Autodesk Inventor part; units mm, degrees
ref_plane "YZ Plane" through (0, 0, 0) normal (1, 0, 0) x (0, 1, 0)
ref_plane "XZ Plane" through (0, 0, 0) normal (0, 1, 0) x (-1, 0, 0)
ref_plane "XY Plane" through (0, 0, 0) normal (0, 0, 1) x (1, 0, 0)
sketch "Sketch1" plane through (0, 0, 0) normal (0, 0, 1) x (1, 0, 0)
  line L0 (-216.5289, 82.2753) -> (-216.5289, 432.2753)
  line L1 (-216.5289, 432.2753) -> (283.4711, 432.2753)
  line L2 (283.4711, 432.2753) -> (283.4711, 82.2753)
  arc A0 (-216.5289, 82.2753) -> (283.4711, 82.2753) centre (33.4711, 82.2753) ccw
  point P0 (0, 0)
  dimension "d0" = 500
  dimension "d1" = 250
  dimension "d2" = 350
extrude "Extrusion1" add sketch "Sketch1" against normal blind 1000
shell "Shell1" thickness 20 removed faces 1 at (-49.8623, 432.2753, -333.3333)
ref_plane "Work Plane1" through (-216.5289, -262.4747, 0) normal (0, 1, 0) x (-1, 0, 0)
sketch "Sketch2" plane through (-216.5289, -262.4747, 0) normal (0, 1, 0) x (-1, 0, 0)
  point P0 (-216.5289, 0)
sketch "Sketch3" plane through (-216.5289, -262.4747, 0) normal (0, 1, 0) x (-1, 0, 0)
  line L0 (-110, -915) -> (-30, -915)
  line L1 (-30, -915) -> (-30, -835)
  line L2 (-30, -835) -> (-110, -835)
  line L3 (-110, -835) -> (-110, -915)
  line L4 (-390, -915) -> (-470, -915)
  line L5 (-470, -915) -> (-470, -835)
  line L6 (-470, -835) -> (-390, -835)
  line L7 (-390, -835) -> (-390, -915)
  line L8 (-500, 0) -> (-500, -1000)
  line L9 (0, 0) -> (0, -1000)
  line L10 (-500, -1000) -> (0, -1000)
  line L11 (0, 0) -> (0, -1000)
  line L12 (0, -500) -> (-564.0368, -500)
  line L13 (-110, -85) -> (-30, -85)
  line L14 (-30, -85) -> (-30, -165)
  line L15 (-110, -165) -> (-110, -85)
  line L16 (-390, -85) -> (-470, -85)
  line L17 (-470, -85) -> (-470, -165)
  line L18 (-470, -165) -> (-390, -165)
  line L19 (-390, -165) -> (-390, -85)
  line L20 (-110, -165) -> (-30, -165)
  point P0 (-216.5289, 0)
  dimension "d6" = 80
  dimension "d7" = 80
  dimension "d8" = 30
  dimension "d10" = 30
  dimension "d11" = 85
extrude "Extrusion2" add sketch "Sketch3" along normal up to next contours L3 L2 L1 L0 | L4 L5 L6 L7 | L13 L14 L20 L15 | L19 L18 L17 L16
sketch "Sketch4" plane through (-216.5289, 432.2753, 0) normal (0, 1, 0) x (1, 0, 0)
  line L0 (14.5, 14.5) -> (485.5, 14.5)
  line L1 (485.5, 14.5) -> (485.5, 985.5)
  line L2 (485.5, 985.5) -> (14.5, 985.5)
  line L3 (14.5, 985.5) -> (14.5, 14.5)
  line L4 (480, 980) -> (480, 20)
  line L5 (480, 20) -> (20, 20)
  line L6 (20, 20) -> (20, 980)
  line L7 (20, 980) -> (480, 980)
  point P0 (216.5289, 0)
  dimension "d14" = 5.5
  dimension "d15" = 5.5
  dimension "d16" = 5.5
  dimension "d17" = 5.5
extrude "Extrusion3" cut sketch "Sketch4" against normal blind 30
properties part number "Composter"
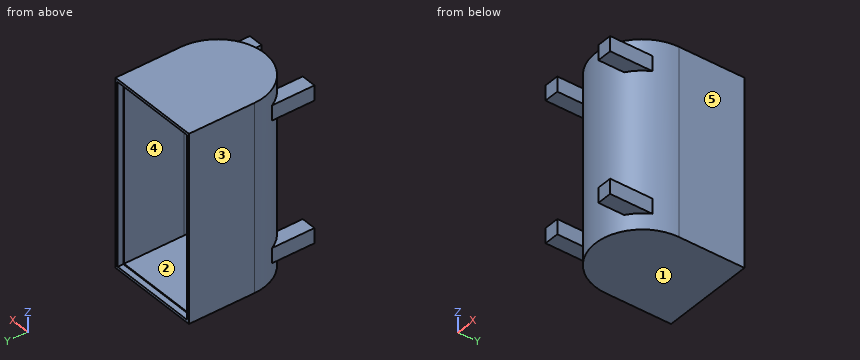
Model file for the job. Use its own axes, mm. Face numbers are marked on the shaded views. A direction names the side the tool comes from. Coordinates: 2 decimals unless noted, no trailing zeros. Write each loop counter-clockwise with the first axis right and the second up, starting at its lowest first coordinate (ties: lowest second). Pieces come first, ordered by that corner, then holes. Notation, with made-up numbers: (79, 71) - (130, 71) arc R6 cw to (130, 78) - close; hole circle Ø7 at (-32.75, 71). An arc over 180 degrees is marked (long way). One line per item, written item: value. Start each with the question number.
1. Slice it at C-C (y = 199). Write the cut outline in (x, z).
2. Flat gauge pins, fed straight in: pin 1 (24 mm diameter, centred on y = -136, z = -892.5, fed in from +X); pin 2 (6 mm diameter, centred on y = -85.5, z = -334, fed in from -X); pin 3 (24 mm diameter, centred on x = 202, y = -204.5, fed in from +Z). Where does each tip first touch, or does it go through?
3. Mould opens along X. For the marked faces 1, 2 and 3 say: released by +X, released by -X, zero draft, split by the parting line, or undercut.
4. Probe line 1 (X direction, y = 144, z = -907); line 2 (Z direction, x = 244.5, y = -56.5); line 3 (Z direction, x = -20, y = 340). List the from-to ranges inside material, lowest first. Write a range as from..to.
5. Slice it at B-B (z = -146). Write the cut outline in (x, y).
6. Slice it at D-D (x = 60.5). Write the cut outline in (y, z).
7. Tool access for the marked faces 4 and 5: list every direction of +Z, -Z, +X, -X, +Y, -Y with a clear straight run to the whole face (end or side of a thin tool).
8. Slice it at A-A (y = -186). Write the cut outline in (x, z), plus the area to 3 significant figures.
Answers below:
1. outline: (-216.53, -1000) - (283.47, -1000) - (283.47, 0) - (-216.53, 0) - close; hole (-196.53, -980) - (263.47, -980) - (263.47, -20) - (-196.53, -20) - close
2. pin 1: stops at x = 253.47
2. pin 2: stops at x = -154.54
2. pin 3: stops at z = -85
3. face 1: zero draft
3. face 2: undercut
3. face 3: released by -X
4. line 1: x = -216.53..-196.53, 263.47..283.47
4. line 2: z = -915..-835, -165..-85
4. line 3: z = -1000..-980, -20..0
5. outline: (-216.53, 82.28) arc R250 ccw to (-186.53, -36.47) - (-186.53, -262.47) - (-106.53, -262.47) - (-106.53, -124.85) arc R250 ccw to (173.47, -124.85) - (173.47, -262.47) - (253.47, -262.47) - (253.47, -36.47) arc R250 ccw to (283.47, 82.28) - (283.47, 432.28) - (268.97, 432.28) - (268.97, 402.28) - (263.47, 402.28) - (263.47, 82.28) arc R230 cw to (-196.53, 82.28) - (-196.53, 402.28) - (-202.03, 402.28) - (-202.03, 432.28) - (-216.53, 432.28) - close
6. outline: (-166.26, -1000) - (432.28, -1000) - (432.28, -985.5) - (402.28, -985.5) - (402.28, -980) - (-146.13, -980) - (-146.13, -20) - (402.28, -20) - (402.28, -14.5) - (432.28, -14.5) - (432.28, 0) - (-166.26, 0) - close
7. face 4: +Y
7. face 5: +Z, -Z, +X, +Y, -Y
8. outline: (-186.53, -915) - (-106.53, -915) - (-106.53, -835) - (-186.53, -835) - close; (-186.53, -165) - (-106.53, -165) - (-106.53, -85) - (-186.53, -85) - close; (173.47, -915) - (253.47, -915) - (253.47, -835) - (173.47, -835) - close; (173.47, -165) - (253.47, -165) - (253.47, -85) - (173.47, -85) - close
8. area: 25,600 mm^2
